Model file for the job. Use its own axes, mm. Face numbers are marked on the shaded views. Round coordinates to 2 decimals unless told otherwise and drop trailing zeros. Loops run counter-clockwise (first coordinate to the right, second up) from the corner with the lowest first, then second, coordinate; pieces in that order, holes last. Notation, with made-up numbers: M 12.5,32 L 29.5,32 A25 cw 29.5,66 Z; hole C 37,9.25 d7. An arc over 180 degrees is marked long. Use a Markdown table: item, result. Add a question column.
Q1. Pin check, flat tip, straight feed: pin 1 (2 mm diameter, centred on y = 10, z = 38.5, fed in from +X). Stop position of the tip, or through.
Q2. Cut at A-A (y = 14). Give the cut face in (x, z), plus the area to 3 significant figures.
Q3. Probe line 1 (Z direction, x = -5.5, y = 16.25); line 2 (Y direction, x = -27, z = 38); line 3 (Z direction, x = -13.75, y = 11.75). List the from-to ranges inside material, lowest first. Write a range as from..to.
Q4. Cut at B-B (z = 33.5). Give the cut face in (x, y), plus the area to 3 significant figures.
Q5. Mould opens along Y. For the marked faces 1, 2, 3 and 4 say: +Y half, -Y half, draft (parallel to the pull), parting line (faces both ways), or undercut.
Q6. Cut at C-C (x = -11.5). Give the cut face in (y, z), plus the area to 3 significant figures.
from build123d import *

# Parameters (mm, degrees)
F0_W       = 29.4857565314
F0_H       = 24.8636654578
F1_DEPTH   = 64.262
F2_R       = 6.0488126263
F1_FACE1_W = 24.8636654578
F1_FACE1_H = 64.262
F3_DEPTH   = 36.322


with BuildPart() as f1:
    # F0 (on Top) → F1 (new body)
    with BuildSketch(Plane.XY):
        with Locations((-14.7428782657, 16.4960857946)):
            Rectangle(F0_W, F0_H)
    extrude(amount=F1_DEPTH)

    # F2 (on face) + F1_face1 (on face) → F3 (cut)
    with BuildSketch(Plane(origin=(-29.4857565314, 0, 0), x_dir=(0, -1, 0), z_dir=(-1, 0, 0))):
        with Locations((-16.0558279604, 34.5874093473)):
            Circle(F2_R)
    with BuildSketch(Plane(origin=(0, 16.4960857946, 32.131), x_dir=(0, 1, 0), z_dir=(1, 0, 0))):
        Rectangle(F1_FACE1_W, F1_FACE1_H)
    extrude(amount=-F3_DEPTH, dir=(-1, 0, 0), mode=Mode.SUBTRACT)


solid = f1.part
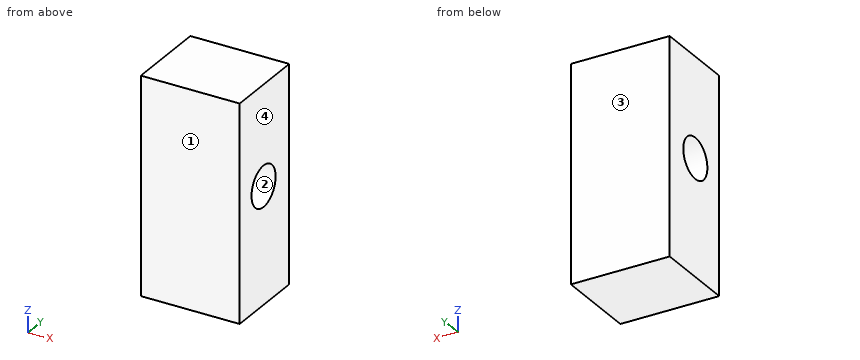
Checked values:
| question | item | result |
|---|---|---|
| 1 | pin 1 | stops at x = 0 |
| 2 | outline | M -29.49,0 L 0,0 L 0,28.9 L -29.49,28.9 Z; M -29.49,40.28 L 0,40.28 L 0,64.26 L -29.49,64.26 Z |
| 2 | area | 1,560 mm^2 |
| 3 | line 1 | z = 0..28.54, 40.63..64.26 |
| 3 | line 2 | y = 4.06..11.06, 21.05..28.93 |
| 3 | line 3 | z = 0..30.34, 38.84..64.26 |
| 4 | outline | M -29.49,4.06 L 0,4.06 L 0,10.11 L -29.49,10.11 Z; M -29.49,22.01 L 0,22.01 L 0,28.93 L -29.49,28.93 Z |
| 4 | area | 382 mm^2 |
| 5 | face 1 | -Y half |
| 5 | face 2 | undercut |
| 5 | face 3 | +Y half |
| 5 | face 4 | draft |
| 6 | outline | M 4.06,0 L 28.93,0 L 28.93,64.26 L 4.06,64.26 Z; hole C 16.06,34.59 d12.1 |
| 6 | area | 1,480 mm^2 |
